```python
from build123d import *

# Parameters (mm, degrees)
F0_R     = 19.05
F1_DEPTH = 1.27
F2_R     = 5.08
F3_DEPTH = 2.54
F4_R     = 19.05
F4_R_2   = 5.08
F5_DEPTH = 1.27
F6_R     = 2.54
F7_DEPTH = 25.4
F8_R     = 2.54
F9_DEPTH = 25.4


with BuildPart() as f1:
    # F0 (on Top) → F1 (new body)
    with BuildSketch(Plane.XY):
        Circle(F0_R)
    extrude(amount=F1_DEPTH)

    # F2 (on face) → F3 (join)
    with BuildSketch(Plane.XY.offset(1.27)):
        Circle(F2_R)
    extrude(amount=F3_DEPTH)

    # F4 (on face) → F5 (join)
    with BuildSketch(Plane.XY.offset(3.81)):
        Circle(F4_R)
        Circle(F4_R_2, mode=Mode.SUBTRACT)
        Circle(F4_R_2)
    extrude(amount=F5_DEPTH)

    # F6 (on face) → F7 (cut)
    with BuildSketch(Plane.XY.offset(5.08)):
        Circle(F6_R)
    extrude(amount=-F7_DEPTH, mode=Mode.SUBTRACT)

    # F8 (on face) → F9 (cut)
    with BuildSketch(Plane.XY.offset(5.08)):
        with BuildLine():
            ThreePointArc((0, 10.16), (1.7960512242, 10.9039487758), (2.54, 12.7))
            ThreePointArc((2.54, 12.7), (-1.7960512242, 14.4960512242), (0, 10.16))
        make_face()
        with BuildLine():
            ThreePointArc((15.24, 0), (12.7, 2.54), (10.16, 0))
            ThreePointArc((10.16, 0), (12.7, -2.54), (15.24, 0))
        make_face()
        with BuildLine():
            ThreePointArc((2.54, -12.7), (1.7960512242, -10.9039487758), (0, -10.16))
            ThreePointArc((0, -10.16), (-1.7960512242, -14.4960512242), (2.54, -12.7))
        make_face()
        with Locations((-12.7, 0)):
            Circle(F8_R)
    extrude(amount=-F9_DEPTH, mode=Mode.SUBTRACT)


solid = f1.part
```
Geometry check sheet. Reference: the model listing, model coordinates, mm. A direction names the side the tool comes from. Coordinates: 2 decimals unless noted, no trailing zeros. Loops run counter-clockwise (first coordinate to the right, second up) from the corner with the lowest first, then second, coordinate; pieces in that order, holes last. Notation, with made-up numbers: (57.5, 66) -> (66.5, 66) arc R19 ccw to (66.5, 103) -> close; hole circle Ø3 at (43.5, 66.5). An arc over 180 degrees is marked (long way). Put each result on its own line as item: value.
1) Gauge pin test, flat ends, axial feed: pin 1 Ø1.5 at (y, z) = (13.5, 4.5) entering from +X; pin 2 Ø1 at (x, z) = (-5, 3) entering from -Y; pin 3 Ø4 at (x, y) = (0, -12.7) entering from -Z; pin 4 Ø2 at (x, z) = (-6.5, 3) entering from -Y. Record the tip position at first contact, or that the pin passes through.
Result set:
pin 1: stops at x = 14.15
pin 2: stops at y = -2.36
pin 3: passes through
pin 4: stops at y = -18.11
2) Cross-section at D-D on y = -8.5. Record the boundary of the cut face in (x, z).
Result set:
outline: (-17.05, 0) -> (17.05, 0) -> (17.05, 1.27) -> (-17.05, 1.27) -> close; (-17.05, 3.81) -> (17.05, 3.81) -> (17.05, 5.08) -> (-17.05, 5.08) -> close
3) Release check for a two-part mould opening along Z. For faces 3 (the flat face through (4, -4, 1.27)), 4 (the cylindrical face through (-0.661, 5.037, 2.522)), 5 (the flat face through (4, 0, 5.08)), 6 (the cylindrical face through (-15.238, 0.112, 0.644)) record: released by +Z, released by -Z, zero draft, split by the parting line, or undercut.
Result set:
face 3: undercut
face 4: undercut
face 5: released by +Z
face 6: zero draft
4) Thickness scan on line 1 (Z direction, x = 9.5, y = -1); line 2 (Y direction, x = 12.7, z = 4.15); line 3 (X direction, y = -2, z = 4.35). Record the ranges inside material, lowest first.
Result set:
line 1: z = 0 to 1.27, 3.81 to 5.08
line 2: y = -14.2 to -2.54, 2.54 to 14.2
line 3: x = -18.94 to -14.27, -11.13 to -1.57, 1.57 to 11.13, 14.27 to 18.94
5) Cross-section at B-B on x = -12. Record the boundary of the cut face in (y, z).
Result set:
outline: (-14.8, 0) -> (-2.44, 0) -> (-2.44, 1.27) -> (-14.8, 1.27) -> close; (-14.8, 3.81) -> (-2.44, 3.81) -> (-2.44, 5.08) -> (-14.8, 5.08) -> close; (2.44, 0) -> (14.8, 0) -> (14.8, 1.27) -> (2.44, 1.27) -> close; (2.44, 3.81) -> (14.8, 3.81) -> (14.8, 5.08) -> (2.44, 5.08) -> close
6) Cross-section at C-C on z = 0.5. Record the boundary of the cut face in (x, y).
Result set:
outline: circle Ø38.1 at (0, 0); hole circle Ø5.08 at (-12.7, 0); hole circle Ø5.08 at (0, -12.7); hole circle Ø5.08 at (0, 0); hole circle Ø5.08 at (0, 12.7); hole circle Ø5.08 at (12.7, 0)
7) Cross-section at A-A on y = 0. Count the separate pieces of the cut face and the enclosed holes in it, plus the area to 3 significant figures.
Result set:
separate pieces: 6
enclosed holes: 0
area: 71.0 mm^2
8) Tool access check on faces 1 (the flat face through (4, 0, 0)), 2 (the flat face through (4, -4, 3.81)). Record the directions out of +Z, -Z, +X, -X, +Y, -Y that give a thin tool (end or side, any length) a straight path to the whole face; none if there is none.
Result set:
face 1: -Z, +X, -X, +Y, -Y
face 2: none
